Work out the finished part from the listing and answer in its coordinate system (mm). Face numbers are marked on the shaded views. A direction names the side the tool comes from. Round coordinates to 2 decimals unless told otherwise and drop trailing zeros. Write each loop counter-clockwise with the first axis right and the second up, starting at its lowest first coordinate (ties: lowest second). Pieces come first, ordered by that corner, then holes.
from build123d import *

# Parameters (mm, degrees)
CUT_EXTRUDE1_DEPTH      = 31.199528082
CUT_EXTRUDE1_DEPTH_BACK = 31.199528082
SKETCH2_W               = 6
SKETCH2_H               = 12
BOSS_EXTRUDE1_DEPTH     = 3.5
CUT_EXTRUDE4_DEPTH      = 45.463597463
CUT_EXTRUDE4_DEPTH_BACK = 15
SKETCH4_W               = 0.806252715
SKETCH4_H               = 7
CUT_EXTRUDE5_DEPTH      = 14
CUT_EXTRUDE5_DEPTH_BACK = 14
SKETCH5_R               = 1.5
CUT_EXTRUDE6_DEPTH      = 12
CUT_EXTRUDE7_START      = 10
CUT_EXTRUDE7_DEPTH      = 18
SKETCH8_R               = 1
CUT_EXTRUDE8_DEPTH      = 45.463597463
SKETCH9_R               = 1


with BuildPart() as part:
    # Sketch1 → Revolve1 (revolve)
    with BuildSketch(Plane(origin=(0, 0, 0), x_dir=(0, 0, -1), z_dir=(1, 0, 0))):
        with BuildLine():
            Line((0, 0), (0, 28))
            Line((0, 28), (5.5, 28))
            add(Edge.make_bspline(
                [(5.5, 28), (8.088190451, 18.340741737), (8, 3.333333333), (8, 0)],
                knots=[0, 0, 0, 0, 1, 1, 1, 1], degree=3))
            Line((8, 0), (0, 0))
        make_face()
    revolve(axis=Axis((0, 0, 0), (0, 1, 0)))

    # Sketch2 → Cut-Extrude1 (cut, two sides: drawn at the far end of the back side and taken through both)
    with BuildSketch(Plane(origin=(0, 0, 0), x_dir=(0, 0, -1), z_dir=(1, 0, 0)).offset(-CUT_EXTRUDE1_DEPTH_BACK)):
        with Locations((0, 22)):
            Rectangle(SKETCH2_W, SKETCH2_H)
    extrude(amount=CUT_EXTRUDE1_DEPTH + CUT_EXTRUDE1_DEPTH_BACK, mode=Mode.SUBTRACT)

    # Sketch3 → Boss-Extrude1 (add, symmetric)
    with BuildSketch(Plane.XY):
        with BuildLine():
            Line((-8, 0), (-8, -15))
            Line((-8, -15), (0, -15))
            ThreePointArc((0, -15), (5.656854249, -12.656854249), (8, -7))
            Line((8, -7), (8, 0))
            Line((8, 0), (-8, 0))
        make_face()
    extrude(amount=BOSS_EXTRUDE1_DEPTH, both=True)

    # Sketch4 → Cut-Extrude4 (cut, two sides: drawn at the far end of the back side and taken through both)
    with BuildSketch(Plane.XZ.offset(15).offset(-CUT_EXTRUDE4_DEPTH_BACK)):
        with Locations((-7.596873643, 0)):
            Rectangle(SKETCH4_W, SKETCH4_H)
        with Locations((7.596873643, 0)):
            Rectangle(SKETCH4_W, SKETCH4_H)
    extrude(amount=CUT_EXTRUDE4_DEPTH + CUT_EXTRUDE4_DEPTH_BACK, mode=Mode.SUBTRACT)

    # Sketch5 → Cut-Extrude5 (cut, two sides: drawn at the far end of the back side and taken through both)
    with BuildSketch(Plane.XY.offset(-CUT_EXTRUDE5_DEPTH_BACK)):
        with Locations(Location((0, 23, 0), (0, 0, 270))):
            Circle(SKETCH5_R)
        with Locations((0, -10)):
            Circle(SKETCH5_R)
    extrude(amount=CUT_EXTRUDE5_DEPTH + CUT_EXTRUDE5_DEPTH_BACK, mode=Mode.SUBTRACT)

    # Sketch6 → Cut-Extrude6 (cut)
    with BuildSketch(Plane(origin=(0, 16, 0), x_dir=(1, 0, 0), z_dir=(0, 1, 0))):
        with BuildLine():
            ThreePointArc((-4.500600684, 3), (-5.408826723, 0), (-4.500600684, -3))
            Line((-4.500600684, -3), (4.500600684, -3))
            ThreePointArc((4.500600684, -3), (5.176793204, -1.567232795), (5.408826723, 0))
            ThreePointArc((5.408826723, 0), (5.176793204, 1.567232795), (4.500600684, 3))
            Line((4.500600684, 3), (-4.500600684, 3))
        make_face()
    extrude(amount=-CUT_EXTRUDE6_DEPTH, mode=Mode.SUBTRACT)

    # Sketch7 → Cut-Extrude7 (cut)
    with BuildSketch(Plane.XY.offset(CUT_EXTRUDE7_START)):
        with BuildLine():
            add(Edge.make_bspline(
                [(4.609772229, 28), (4.921871239, 27.023759734), (5.179569274, 26.037706908), (5.483962232, 24.698137834), (5.558895001, 24.349714977), (5.630197487, 24.00063731)],
                knots=[0, 0, 0, 0, 0.25, 0.25, 0.337633548, 0.337633548, 0.337633548, 0.337633548], degree=3))
            Line((4.609772229, 28), (0.731348135, 28))
            ThreePointArc((0.731348135, 28), (3.893373866, 26.873189032), (5.630197487, 24.00063731))
        make_face()
        with BuildLine():
            ThreePointArc((-5.630197487, 24.00063731), (-3.893373866, 26.873189032), (-0.731348135, 28))
            Line((-0.731348135, 28), (-4.609772229, 28))
            add(Edge.make_bspline(
                [(-5.630197487, 24.00063731), (-5.558895001, 24.349714977), (-5.483962232, 24.698137834), (-5.179569274, 26.037706908), (-4.921871239, 27.023759734), (-4.609772229, 28)],
                knots=[0.662366452, 0.662366452, 0.662366452, 0.662366452, 0.75, 0.75, 1, 1, 1, 1], degree=3))
        make_face()
    extrude(amount=-CUT_EXTRUDE7_DEPTH, mode=Mode.SUBTRACT)

    # Sketch8 → Cut-Extrude8 (cut, through all)
    with BuildSketch(Plane.XZ.offset(15)):
        with Locations(Location((3, 0, 0), (0, 0, 270))):
            Circle(SKETCH8_R)
    extrude(amount=-CUT_EXTRUDE8_DEPTH, mode=Mode.SUBTRACT)

    # Cut-Sweep1: sweep along a path in Sketch10
    with BuildLine() as cut_sweep1_path:  # in the path sketch's own coordinates; laid on its plane below (add() does not lay a ready-made edge on the line's plane)
        add(Edge.make_bspline(
            [(-7.193747285, -7.5), (-2.693747285, -7.5), (-2.693747285, 4)],
            knots=[0, 0, 0, 1, 1, 1], degree=2))
    # Sketch9 → Cut-Sweep1 (sweep, cut)
    with BuildSketch(Plane.ZY.offset(7.193747285)):
        with Locations((0, -7.5)):
            Circle(SKETCH9_R)
    sweep(path=Plane.XY * cut_sweep1_path.line, mode=Mode.SUBTRACT)


solid = part.part
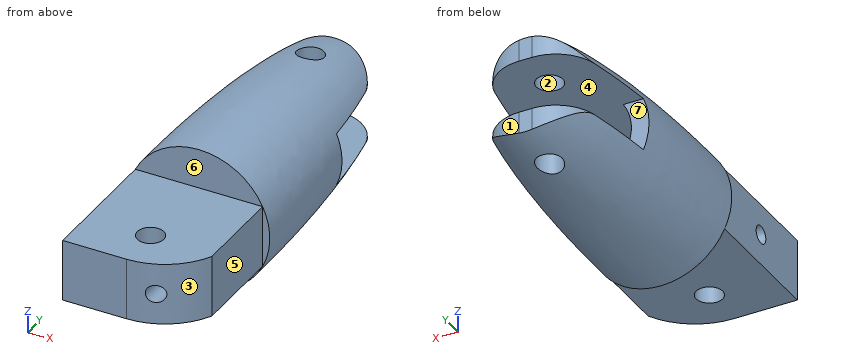
Q1. The mould has two halves that part along Y. Classify the marked faces 1, 2, 3 and 4: +Y half, -Y half, draft (parallel to the pull), parting line (faces both ways), or undercut.
Q2. Given pin 1 (6 mm diameter, centred on x = 4.5, y = -4, fed in from -Z); pin 2 (1.3 mm diameter, centred on x = -1.5, z = 5, fed in from -Y); pin 3 (3 mm diameter, centred on x = 6.5, z = -0.5, fed in from +Y), each flat-ended and moving along its own axis, determine where each tip first touches the part or whether it passes through.
Q3. Find section B-B (y = 23). Count the separate pieces of the cut face and the enclosed holes in it, plus the area to 3 significant figures.
Q4. Find the intervals of material crossed by L1, parallel to Y at x = 0, z = 4.65; L2, parallel to Y at x = 0, z = -0.5; L3, parallel to Z at x = 0.75, y = -2, in increasing order.
Q5. Find section A-A (y = -10). Determine the outline of the cut face in (x, z), plus the area to 3 significant figures.
Q6. A tool of negligible diameter and unlimited length cuts with its end or side. For the marked faces 5, 6 and 7, from which of +Z, -Z, +X, -X, +Y, -Y can it reach the whole face along a straight path? Write none if from no direction.
Report:
1. face 1: +Y half
1. face 2: undercut
1. face 3: -Y half
1. face 4: draft
2. pin 1: stops at z = -3.5
2. pin 2: stops at y = 0
2. pin 3: stops at y = 16
3. separate pieces: 4
3. enclosed holes: 0
3. area: 38.1 mm2
4. L1: y = 0 to 21.5, 24.5 to 28
4. L2: y = -15 to -11.5, -8.5 to 4
4. L3: z = -3.5 to 3.5
5. outline: (-7.19, -3.5) - (-1.5, -3.5) - (-1.5, 3.5) - (-7.19, 3.5) - close; (1.5, -3.5) - (7.19, -3.5) - (7.19, 3.5) - (1.5, 3.5) - close; hole circle Ø2 at (3, 0)
5. area: 76.6 mm2
6. face 5: +Z, -Z, +X, -Y
6. face 6: +Z, +X, -X, -Y
6. face 7: +X, -X, +Y
